Can you work these out from the model? Positions are in its coordinate system, mm. Face numbers are marked on the shaded views. Give positions to 0.01 mm unless a question says otherwise; leave off trailing zeros. Write each loop counter-clockwise with the first axis right and the second up, starting at its lowest first coordinate (ties: lowest second). Pieces come first, ordered by that corner, then holes. Notation, with made-up numbers: M 17,42 L 31,42 A29 cw 31,73 Z; hole C 13.5,34 d2. An arc over 180 degrees is marked long. Answer as CSV lines item,"result". Start each with the question number.
```python
from build123d import *

# Parameters (mm, degrees)
SKETCH1_R                 = 22.225
SKETCH1_R_2               = 20.574
BOSS_EXTRUDE1_DEPTH       = 38.1
SKETCH2_R                 = 2.54
CUT_EXTRUDE1_DEPTH        = 50.8
SKETCH3_R                 = 3.875
SKETCH3_R_2               = 2.25
CUT_EXTRUDE2_DEPTH        = 0.5
SKETCH3_2_R               = 2.25
CUT_EXTRUDE3_DEPTH        = 16.17
CIRPATTERN1_COUNT         = 4
MIRROR1_COPY_1_SKETCH_R   = 3.875
MIRROR1_COPY_1_SKETCH_R_2 = 2.25
MIRROR1_COPY_1_DEPTH      = 0.5
MIRROR1_COPY_2_SKETCH_R   = 3.875
MIRROR1_COPY_2_SKETCH_R_2 = 2.25
MIRROR1_COPY_2_DEPTH      = 0.5
MIRROR1_COPY_3_SKETCH_R   = 3.875
MIRROR1_COPY_3_SKETCH_R_2 = 2.25
MIRROR1_COPY_3_DEPTH      = 0.5
MIRROR1_COPY_4_SKETCH_R   = 2.25
MIRROR1_COPY_4_DEPTH      = 16.17
MIRROR1_COPY_5_SKETCH_R   = 2.25
MIRROR1_COPY_5_DEPTH      = 16.17
MIRROR1_COPY_6_SKETCH_R   = 2.25
MIRROR1_COPY_6_DEPTH      = 16.17


with BuildPart() as part:
    # Sketch1 → Boss-Extrude1 (new body)
    with BuildSketch(Plane(origin=(0, 0, 0), x_dir=(-1, 0, 0), z_dir=(0, 1, 0))):
        with Locations(Location((0, 0, 0), (0, 0, 270))):
            Circle(SKETCH1_R)
        with Locations(Location((0, 0, 0), (0, 0, 270))):
            Circle(SKETCH1_R_2, mode=Mode.SUBTRACT)
    extrude(amount=BOSS_EXTRUDE1_DEPTH)

    # Sketch2 → Cut-Extrude1 (cut)
    with BuildSketch(Plane.YZ):
        with Locations(Location((9.525, 9.525, 0), (0, 0, 90))):
            Circle(SKETCH2_R)
    extrude(amount=CUT_EXTRUDE1_DEPTH, mode=Mode.SUBTRACT)

    # Sketch3 → Cut-Extrude2 (cut)
    with BuildSketch(Plane.XY.offset(22.225)):
        with Locations((0, 30.1)):
            Circle(SKETCH3_R)
        with Locations((0, 30.1)):
            Circle(SKETCH3_R_2, mode=Mode.SUBTRACT)
    cut_extrude2 = extrude(amount=-CUT_EXTRUDE2_DEPTH, mode=Mode.SUBTRACT)

    # Sketch3_2 → Cut-Extrude3 (cut)
    with BuildSketch(Plane.XY.offset(22.225)):
        with Locations((0, 30.1)):
            Circle(SKETCH3_2_R)
    cut_extrude3 = extrude(amount=-CUT_EXTRUDE3_DEPTH, mode=Mode.SUBTRACT)

    # CirPattern1: Cut-Extrude2, Cut-Extrude3 ×4 about axis
    cirpattern1_axis = Axis((0, 0, 0), (0, 1, 0))
    add([cut_extrude2.rotate(cirpattern1_axis, i * 360 / CIRPATTERN1_COUNT) for i in range(1, CIRPATTERN1_COUNT)], mode=Mode.SUBTRACT)
    add([cut_extrude3.rotate(cirpattern1_axis, i * 360 / CIRPATTERN1_COUNT) for i in range(1, CIRPATTERN1_COUNT)], mode=Mode.SUBTRACT)

    # Mirror1: Cut-Extrude2, Cut-Extrude3 across plane
    add(cut_extrude2.mirror(Plane(origin=(0, 19.05, 0), x_dir=(0, 0, 1), z_dir=(0, -1, 0))), mode=Mode.SUBTRACT)
    add(cut_extrude3.mirror(Plane(origin=(0, 19.05, 0), x_dir=(0, 0, 1), z_dir=(0, -1, 0))), mode=Mode.SUBTRACT)

    # Mirror1 copy 1 sketch → Mirror1 copy 1 (cut)
    with BuildSketch(Plane(origin=(22.225, 38.1, 0), x_dir=(0, 0, -1), z_dir=(1, 0, 0))):
        with Locations((0, -30.1)):
            Circle(MIRROR1_COPY_1_SKETCH_R)
        with Locations((0, -30.1)):
            Circle(MIRROR1_COPY_1_SKETCH_R_2, mode=Mode.SUBTRACT)
    extrude(amount=-MIRROR1_COPY_1_DEPTH, mode=Mode.SUBTRACT)

    # Mirror1 copy 2 sketch → Mirror1 copy 2 (cut)
    with BuildSketch(Plane(origin=(0, 38.1, -22.225), x_dir=(-1, 0, 0), z_dir=(0, 0, -1))):
        with Locations((0, -30.1)):
            Circle(MIRROR1_COPY_2_SKETCH_R)
        with Locations((0, -30.1)):
            Circle(MIRROR1_COPY_2_SKETCH_R_2, mode=Mode.SUBTRACT)
    extrude(amount=-MIRROR1_COPY_2_DEPTH, mode=Mode.SUBTRACT)

    # Mirror1 copy 3 sketch → Mirror1 copy 3 (cut)
    with BuildSketch(Plane(origin=(-22.225, 38.1, 0), x_dir=(0, 0, 1), z_dir=(-1, 0, 0))):
        with Locations((0, -30.1)):
            Circle(MIRROR1_COPY_3_SKETCH_R)
        with Locations((0, -30.1)):
            Circle(MIRROR1_COPY_3_SKETCH_R_2, mode=Mode.SUBTRACT)
    extrude(amount=-MIRROR1_COPY_3_DEPTH, mode=Mode.SUBTRACT)

    # Mirror1 copy 4 sketch → Mirror1 copy 4 (cut)
    with BuildSketch(Plane(origin=(22.225, 38.1, 0), x_dir=(0, 0, -1), z_dir=(1, 0, 0))):
        with Locations((0, -30.1)):
            Circle(MIRROR1_COPY_4_SKETCH_R)
    extrude(amount=-MIRROR1_COPY_4_DEPTH, mode=Mode.SUBTRACT)

    # Mirror1 copy 5 sketch → Mirror1 copy 5 (cut)
    with BuildSketch(Plane(origin=(0, 38.1, -22.225), x_dir=(-1, 0, 0), z_dir=(0, 0, -1))):
        with Locations((0, -30.1)):
            Circle(MIRROR1_COPY_5_SKETCH_R)
    extrude(amount=-MIRROR1_COPY_5_DEPTH, mode=Mode.SUBTRACT)

    # Mirror1 copy 6 sketch → Mirror1 copy 6 (cut)
    with BuildSketch(Plane(origin=(-22.225, 38.1, 0), x_dir=(0, 0, 1), z_dir=(-1, 0, 0))):
        with Locations((0, -30.1)):
            Circle(MIRROR1_COPY_6_SKETCH_R)
    extrude(amount=-MIRROR1_COPY_6_DEPTH, mode=Mode.SUBTRACT)


solid = part.part
```
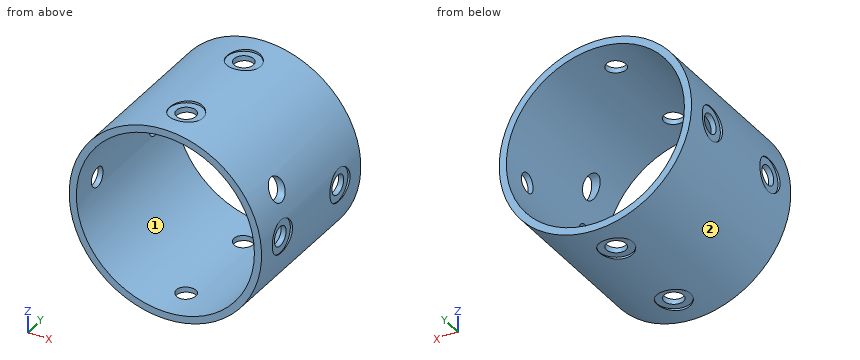
1) I want a section at B-B, the plane z = -10. Please give me the cut outline in (x, y), then the cut area to 3 significant figures.
2) I need wall thicknesses on L1, parallel to Y at x = 0, z = 22 (3 decimals); L2, parallel to Y at x = -21.3, z = 0; L3, parallel to Z at x = -7.5, y = 30. Which ranges of each line are inside material? Lowest first, please. Write a range as from..to.
3) I want a section at D-D, the plane y = 18. Please give me the cut outline in (x, z) (3 decimals).
4) I want a section at C-C, the plane y = 30.1. State how many separate pieces and enclosed holes the cut face has, then the cut area to 3 significant figures.
5) I'm going to push flat-ended pins straight in: P1, Ø7, axis at y = 30.1, z = 0, coming from the +X side (3 decimals); P2, Ø2.5, axis at y = 30.5, z = -0.5, coming from the +X side; P3, Ø7, axis at x = 0, y = 8, coming from the +Z side (3 decimals); P4, Ø7, axis at x = 0, y = 30.1, coming from the -Z side (3 decimals). Where does each tip first touch, or does it pass through?
6) I want a section at A-A, the plane x = 7. Please give me the cut outline in (y, z).
7) Thinking about a two-plate mould opening in X: for the marked faces 1 and 2, which applies, released by +X, released by -X, zero draft, split by the parting line, or undercut?
Values found:
1,outline,"M -19.85,0 L -17.98,0 L -17.98,38.1 L -19.85,38.1 Z; M 17.98,0 L 19.85,0 L 19.85,38.1 L 17.98,38.1 Z"
1,area,"142 mm²"
2,L1,"y = 0..4.125, 11.875..26.225, 33.975..38.1"
2,L2,"y = 0..5.75, 10.25..27.85, 32.35..38.1"
2,L3,"z = -20.92..-19.16, 19.16..20.92"
3,outline,"C 0,0 d44.45; hole C 0,0 d41.148"
4,separate pieces,"4"
4,enclosed holes,"0"
4,area,"189 mm²"
5,P1,"stops at x = 21.725"
5,P2,"passes through"
5,P3,"stops at z = 21.725"
5,P4,"stops at z = -21.725"
6,outline,"M 0,-21.09 L 38.1,-21.09 L 38.1,-19.35 L 0,-19.35 Z; M 0,19.35 L 38.1,19.35 L 38.1,21.09 L 0,21.09 Z"
7,face 1,"undercut"
7,face 2,"split by the parting line"
